Work out the finished part from the listing and answer in its coordinate system (mm). A direction names the side the tool comes from. Round coordinates to 2 decimals unless told otherwise and drop trailing zeros. Write each loop counter-clockwise with the first axis right and the second up, starting at its lowest first coordinate (ties: lowest second). Pieces come first, ordered by that corner, then holes. Notation, with made-up numbers: M -28.5,78 L 2.5,78 A29 ccw 2.5,113 Z; hole C 59.25,-19 d8. An arc over 180 degrees is marked long. Answer in a Markdown table with one row per item.
```python
from build123d import *

# Parameters (mm, degrees)
EXTRUDE_1_DEPTH          = 30
SKETCH_2_W               = 80
SKETCH_2_H               = 60
EXTRUDE_2_DEPTH          = 20
FILLET_1_R               = 10
SKETCH_3_W               = 60
SKETCH_3_H               = 20
CUT_EXTRUDE_1_DEPTH      = 124.693168769
SKETCH_4_W               = 110
SKETCH_4_H               = 80
EXTRUDE_3_DEPTH          = 60
CUT_EXTRUDE_2_DEPTH      = 193.418814049
SKETCH_6_W               = 158
SKETCH_6_H               = 100
SKETCH_6_W_2             = 110
SKETCH_6_H_2             = 63.245553204
EXTRUDE_4_DEPTH          = 15
FILLET_2_R               = 20
CUT_EXTRUDE_3_DEPTH      = 3
CUT_EXTRUDE_4_DEPTH      = 212.765112606
CUT_EXTRUDE_4_DEPTH_BACK = 212.765112606
SKETCH_8_W               = 52
SKETCH_8_H               = 56


with BuildPart() as part:
    # 草图1 → 凸台-拉伸1 (new, symmetric)
    with BuildSketch(Plane.XY):
        Polygon((-40, 40), (-90, 0), (-30, 0), (-30, 10), (30, 10), (30, 0), (90, 0), (40, 40), align=None)
    extrude(amount=EXTRUDE_1_DEPTH, both=True)

    # 草图2 → 凸台-拉伸2 (add)
    with BuildSketch(Plane(origin=(0, 40, 0), x_dir=(1, 0, 0), z_dir=(0, 1, 0))):
        Rectangle(SKETCH_2_W, SKETCH_2_H)
    extrude(amount=EXTRUDE_2_DEPTH)

    # 圆角1
    fillet_1_edges = [part.edges().sort_by_distance(p)[0] for p in [
        (40, 40, 0),
        (-40, 40, 0),
    ]]
    fillet(fillet_1_edges, radius=FILLET_1_R)

    # 草图3 → 切除-拉伸1 (cut, through all)
    with BuildSketch(Plane.XY.offset(30)):
        with Locations((0, 50)):
            Rectangle(SKETCH_3_W, SKETCH_3_H)
    extrude(amount=-CUT_EXTRUDE_1_DEPTH, mode=Mode.SUBTRACT)

    # 草图4 → 凸台-拉伸3 (add)
    with BuildSketch(Plane(origin=(0, 60, 0), x_dir=(1, 0, 0), z_dir=(0, 1, 0))):
        Rectangle(SKETCH_4_W, SKETCH_4_H)
    extrude(amount=EXTRUDE_3_DEPTH)

    # 草图5 → 切除-拉伸2 (cut, through all)
    with BuildSketch(Plane.ZY.offset(55)):
        Polygon((20, 120), (40, 60), (40, 120), align=None)
    extrude(amount=-CUT_EXTRUDE_2_DEPTH, mode=Mode.SUBTRACT)

    # 草图6 → 凸台-拉伸4 (add)
    # profile 1 of 2: a face of its own
    with BuildSketch(Plane(origin=(0, 18, 54), x_dir=(1, 0, 0), z_dir=(0, 0.31622776601683805, 0.9486832980505138))):
        with Locations((0, 75.894663844)):
            Rectangle(SKETCH_6_W, SKETCH_6_H)
        with Locations((0, 75.894663844)):
            Rectangle(SKETCH_6_W_2, SKETCH_6_H_2, mode=Mode.SUBTRACT)
    # profile 2 of 2: a face of its own
    with BuildSketch(Plane(origin=(0, 18, 54), x_dir=(1, 0, 0), z_dir=(0, 0.31622776601683805, 0.9486832980505138))):
        with Locations((0, 75.894663844)):
            Rectangle(SKETCH_6_W_2, SKETCH_6_H_2)
    extrude(amount=EXTRUDE_4_DEPTH)

    # 圆角2
    fillet_2_edges = [part.edges().sort_by_distance(p)[0] for p in [
        (-79, 44.937543343, 52.926513036),
        (79, 44.937543343, 52.926513036),
        (79, 139.805873148, 21.303736435),
        (-79, 139.805873148, 21.303736435),
    ]]
    fillet(fillet_2_edges, radius=FILLET_2_R)

    # 草图7 → 切除-拉伸3 (cut)
    with BuildSketch(Plane(origin=(0, 22.74341649, 68.230249471), x_dir=(1, 0, 0), z_dir=(0, 0.3162277660168381, 0.9486832980505138))):
        with BuildLine():
            Line((69, 45.894663844), (69, 105.894663844))
            ThreePointArc((69, 105.894663844), (66.071067812, 112.965731656), (59, 115.894663844))
            Line((59, 115.894663844), (-59, 115.894663844))
            ThreePointArc((-59, 115.894663844), (-66.071067812, 112.965731656), (-69, 105.894663844))
            Line((-69, 105.894663844), (-69, 45.894663844))
            ThreePointArc((-69, 45.894663844), (-66.071067812, 38.823596032), (-59, 35.894663844))
            Line((-59, 35.894663844), (59, 35.894663844))
            ThreePointArc((59, 35.894663844), (66.071067812, 38.823596032), (69, 45.894663844))
        make_face()
    extrude(amount=-CUT_EXTRUDE_3_DEPTH, mode=Mode.SUBTRACT)

    # 草图8 → 切除-拉伸4 (cut, two sides: drawn at the far end of the back side and taken through both)
    with BuildSketch(Plane(origin=(55, 0, 0), x_dir=(0, 0, -1), z_dir=(1, 0, 0)).offset(-CUT_EXTRUDE_4_DEPTH_BACK)):
        with Locations((0, 32)):
            Rectangle(SKETCH_8_W, SKETCH_8_H)
    extrude(amount=CUT_EXTRUDE_4_DEPTH + CUT_EXTRUDE_4_DEPTH_BACK, mode=Mode.SUBTRACT)


solid = part.part
```
1. Determine the mould class of faces 5 (the flat face through (-0.826, 44.904, 52.827)), 6 (the flat face through (-1, 25, -26)), 7 (the flat face through (-30, 50, 28)) for opening direction Z: released by +Z, released by -Z, zero draft, split by the parting line, or undercut.
Calculated:
| item | result |
|---|---|
| face 5 | released by +Z |
| face 6 | undercut |
| face 7 | zero draft |
2. The part is cut by section C-C (x = -18). Determine the outline of the cut face in (y, z).
Calculated:
| item | result |
|---|---|
| outline | M 10,-30 L 40,-30 L 40,-26 L 10,-26 Z; M 10,26 L 40,26 L 40,30 L 10,30 Z; M 42.57,45.81 L 60,40 L 60,-40 L 120,-40 L 120,20 L 137.43,14.19 L 142.18,28.42 L 132.69,31.58 L 131.74,28.74 L 55.85,54.03 L 56.8,56.88 L 47.31,60.04 Z |
3. A tool of negligible diameter and unlimited length cuts with its end or side. For faces 1 (the flat face through (40, 52, -28)), 2 (the cylindrical face through (-40.96, 40.53, -28.03)), 3 (the cylindrical face through (65.99, 59.03, 54.57)), 4 (the flat face through (30, 3, 0)), from which of +Z, -Z, +X, -X, +Y, -Y can it reach the whole face along a straight path? Write none if from no direction.
Calculated:
| item | result |
|---|---|
| face 1 | -Z, +X |
| face 2 | -Z, -X |
| face 3 | +Y |
| face 4 | +Z, -Z, -Y |
4. The part is cut by section D-D (x = 73). Determine the outline of the cut face in (y, z).
Calculated:
| item | result |
|---|---|
| outline | M 0,-30 L 13.6,-30 L 13.6,-26 L 4,-26 L 4,26 L 13.6,26 L 13.6,30 L 0,30 Z; M 47.99,44 L 132.01,16 L 136.75,30.23 L 52.73,58.23 Z |
5. Consider line 1 along Y through (x, z) = (40, 10.5); line 2 along Z through (x, y) = (-35.5, 15); line 3 along Y through (x, z) = (10, -12). Determine where each line is inside the solid, lowest interval first. Write a range as from..to.
Calculated:
| item | result |
|---|---|
| line 1 | y = 0..4, 60..120 |
| line 2 | z = -30..-26, 26..30 |
| line 3 | y = 60..120 |
6. The part is cut by section A-A (z = 11). Determine the outline of the cut face in (x, y).
Calculated:
| item | result |
|---|---|
| outline | M -90,0 L -30,0 L -30,4 L -85,4 Z; M -55,60 L 55,60 L 55,120 L -55,120 Z; M 30,0 L 90,0 L 85,4 L 30,4 Z |
7. Given pin 1 (1.2 mm diameter, centred on x = 1.5, z = -28, fed in from -Y); pin 2 (10 mm diameter, centred on y = 90.5, z = 38, fed in from +X); pin 3 (2 mm diameter, centred on y = 53.5, z = -28.5, fed in from -X), each flat-ended and moving along its own axis, determine where each tip first touches the part or whether it passes through.
Calculated:
| item | result |
|---|---|
| pin 1 | stops at y = 10 |
| pin 2 | stops at x = 79 |
| pin 3 | stops at x = -40 |
8. The part is cut by section B-B (y = 27). Determine the outline of the cut face in (x, z).
Calculated:
| item | result |
|---|---|
| outline | M -56.25,-30 L 56.25,-30 L 56.25,-26 L -56.25,-26 Z; M -56.25,26 L 56.25,26 L 56.25,30 L -56.25,30 Z |
